Here's the drawing with two shaded views (mm, measured from the low corner). I have some questions. A direction names the side the tool comes from. Coordinates: 2 decimals unless noted, no trailing zeros. Write each loop counter-clockwise with the first axis right and the second up, starting at its lowest first coordinate (ties: lowest second). Pieces come first, ordered by that corner, then holes. Notation, with made-up numbers: M 4,74 L 41,74 A20 cw 41,85 Z; hole C 1.25,42 d2. An arc over 180 degrees is marked long. Answer as CSV lines item,"result". Start each with the question number.
Item 1: We'd pull the mould along Z, two halves only. Please class the marked faces 1, 2 and 3: +Z half, -Z half, draft (parallel to the pull), parting line (faces both ways), or undercut.
Item 2: On a 3-axis mill with a long thin cutter (end or side, diameter ignored), from which of +Z, -Z, +X, -X, +Y, -Y can I reach the whole of each face in a straight line? I mean the marked faces 4 and 5. Say none if no direction works.
Item 3: I'm going to push flat-ended pins straight in: P1, Ø1.5, axis at x = 84, y = 9.5, coming from the -Z side; P2, Ø1.5, axis at x = 46, y = 21, coming from the -Z side; P3, Ø1.5, axis at x = 97.5, y = 22, coming from the +Z side. Where does each tip first touch, or does it pass through?
Item 4: Suppose I cut it at A-A, the plane y = 3.25. Write out the boundary of the cut face in (x, z) (1 decimal).
Item 5: If I drill on line 1 along X through (y, z) = (17, 70.5) (1 decimal); line 2 along X through (y, z) = (18.75, 77.5); line 3 along Y through (x, z) = (40, 15), over which ranges is the centre line in solid material (lowest first)? Write a range as [from, to].
Item 6: Suppose I cut it at B-B, the plane y = 21. Write out the boundary of the cut face in (x, z) (1 decimal), and give its area (3 significant figures).
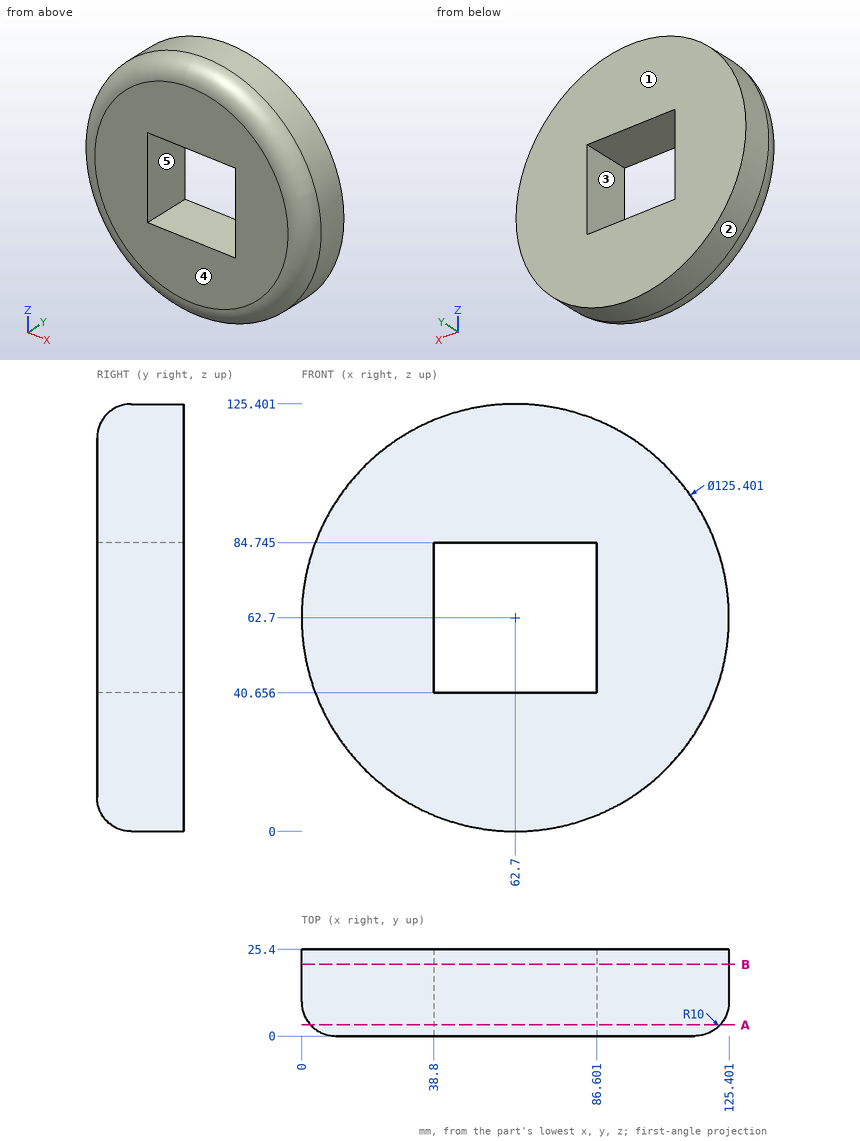
Ans:
1,face 1,"draft"
1,face 2,"parting line"
1,face 3,"undercut"
2,face 4,"+Z, -Z, +X, -X, -Y"
2,face 5,"+Y, -Y"
3,P1,"stops at z = 3.47"
3,P2,"stops at z = 2.06"
3,P3,"stops at z = 115.35"
4,outline,"C 62.7,62.7 d120.2; hole M 38.8,40.7 L 86.6,40.7 L 86.6,84.7 L 38.8,84.7 Z"
5,line 1,"x = [0.5, 38.8], [86.6, 124.9]"
5,line 2,"x = [1.77, 38.8], [86.6, 123.63]"
5,line 3,"y = [0, 25.4]"
6,outline,"C 62.7,62.7 d125.4; hole M 38.8,40.7 L 86.6,40.7 L 86.6,84.7 L 38.8,84.7 Z"
6,area,"10,200 mm^2"
